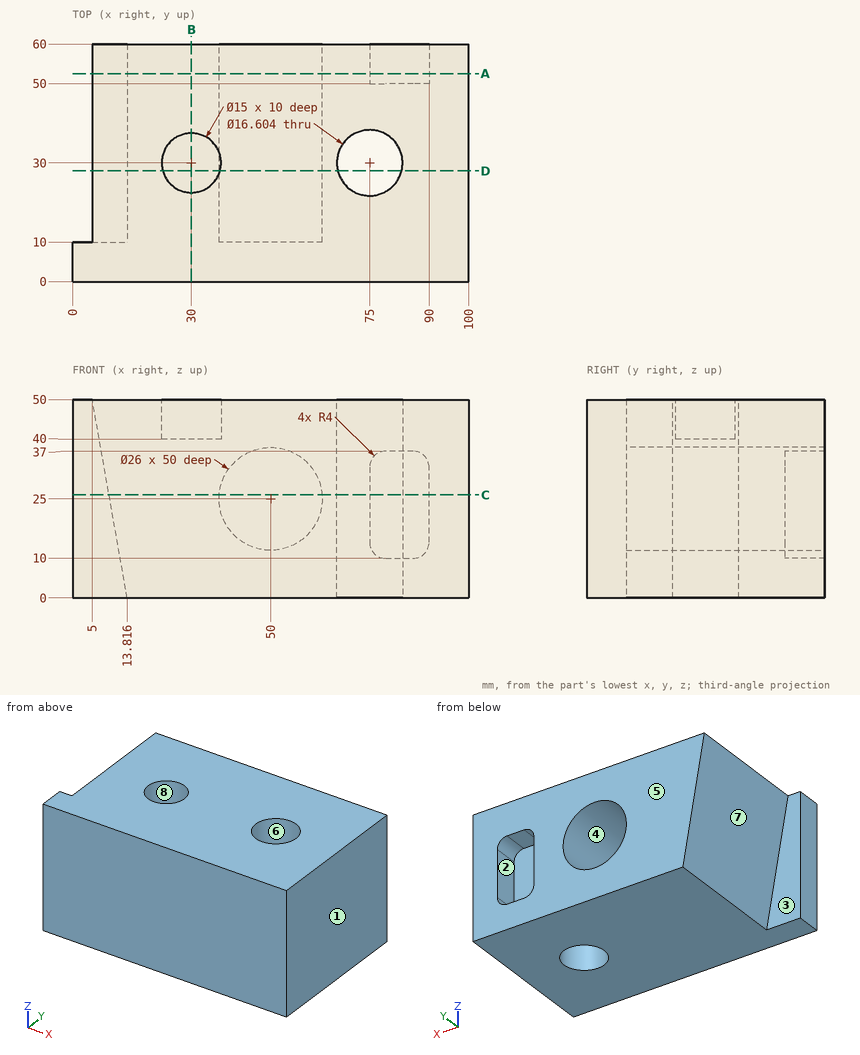
Verification items for this drawing (mm, ordinates from the low corner). A direction names the side the tool comes from. Give positions to 0.01 mm unless a question says otherwise; leave off trailing zeros. Write each loop counter-clockwise with the first axis right and the second up, starting at its lowest first coordinate (ties: lowest second). Pieces come first, ordered by that corner, then holes.
1) Section check C-C, the plane z = 26. Record the boundary of the cut face in (x, y), and give its area (3 significant figures).
2) Section check A-A, the plane y = 52.5. Record the boundary of the cut face in (x, z), and give its area (3 significant figures).
3) Release check for a two-part mould opening along X. For the marked faces 1, 2 and 3 record: pulls with the +X half, pulls with the -X half, needs draft (parallel to the pull), parting line crosses it, or undercut.
4) Material ranges on L1, parallel to X at y = 36.5, z = 44.5 (1 decimal); L2, parallel to X at y = 35, z = 28; L3, parallel to Y at x = 30, z = 45, recorded low to high.
5) Section check D-D, the plane y = 28. Record the boundary of the cut face in (x, z).
6) Gauge pin test, flat ends, axial feed: pin 1 (3 mm diameter, centred on y = 54.5, z = 25, fed in from -X); pin 2 (6 mm diameter, centred on y = 50.5, z = 21.5, fed in from -X); pin 3 (4.5 mm diameter, centred on x = 83, z = 19.5, fed in from +Y); pin 4 (15 mm diameter, centred on x = 75, y = 30, fed in from -Z). Record the tip position at first contact, or that the pin passes through.
7) Section check B-B, the plane x = 30. Record the boundary of the cut face in (y, z), and give its area (3 significant figures).
8) Access from +Z, -Z, +X, -X, +Y, -Y to the whole of each face (thin tool, end or side, straight path). Record for the marked faces 4, 5, 6, 7 and 8.
Computed:
1. outline: (0, 0) - (100, 0) - (100, 60) - (90, 60) - (90, 50) - (75, 50) - (75, 60) - (62.96, 60) - (62.96, 10) - (37.04, 10) - (37.04, 60) - (9.23, 60) - (9.23, 10) - (0, 10) - close; hole circle Ø16.6 at (75, 30)
1. area: 3,880 mm2
2. outline: (5, 50) - (13.82, 0) - (100, 0) - (100, 50) - close; hole circle Ø26 at (50, 25); hole (75, 14) arc R4 ccw to (79, 10) - (86, 10) arc R4 ccw to (90, 14) - (90, 33) arc R4 ccw to (86, 37) - (79, 37) arc R4 ccw to (75, 33) - close
2. area: 3,610 mm2
3. face 1: pulls with the +X half
3. face 2: undercut
3. face 3: needs draft
4. L1: x = 6 to 26.3, 33.7 to 69.8, 80.2 to 100
4. L2: x = 8.88 to 37.35, 62.65 to 68.37, 81.63 to 100
4. L3: y = 0 to 22.5, 37.5 to 60
5. outline: (5, 50) - (13.82, 0) - (66.94, 0) - (66.94, 50) - (37.23, 50) - (37.23, 40) - (22.77, 40) - (22.77, 50) - close; (83.06, 0) - (100, 0) - (100, 50) - (83.06, 50) - close; hole circle Ø26 at (50, 25)
6. pin 1: stops at x = 9.14
6. pin 2: stops at x = 9.5
6. pin 3: stops at y = 50
6. pin 4: passes through
7. outline: (0, 0) - (60, 0) - (60, 50) - (37.5, 50) - (37.5, 40) - (22.5, 40) - (22.5, 50) - (0, 50) - close
7. area: 2,850 mm2
8. face 4: +Y
8. face 5: +Z, -Z, +X, -X, +Y
8. face 6: +Z, -Z
8. face 7: -Z, -X, +Y
8. face 8: +Z
